Can you work these out from the model? Positions are in its coordinate system, mm. A direction names the side the tool comes from. Give positions to 0.01 mm unless a question says otherwise; leave off trailing zeros. Write each loop counter-clockwise with the first axis right and the second up, starting at its lowest first coordinate (ties: lowest second). Pieces come first, ordered by that corner, then holes.
1. On a 3-axis mill with a long thin cutter (end or side, diameter ignored), from which of +Z, -Z, +X, -X, +Y, -Y can I reach the whole of each face in a straight line? I mean faces 4 (the flat face through (-17.77, 4, 31)), 5 (the flat face through (-27.93, 4, 31)), 6 (the flat face through (-23, 1, 34.532)), 7 (the flat face through (-23, -5, 23.737)). Say none if no direction works.
2. Suppose I cut it at D-D (y = 3.81). Please give me the cut outline in (x, z).
3. Suppose I cut it at A-A (y = -4). Please give me the cut outline in (x, z), and give its area (3 significant figures).
4. Suppose I cut it at C-C (z = 28.25). Please give me the cut outline in (x, y), and give its area (3 significant figures).
5. I'm going to push flat-ended pins straight in: pin 1 (2.5 mm diameter, centred on x = -21.5, y = 5, fed in from +Z); pin 2 (1 mm diameter, centred on y = 1, z = 26, fed in from -X); pin 3 (4 mm diameter, centred on x = -21.5, y = 5, fed in from -Z); pin 4 (3 mm diameter, centred on x = -29.5, z = 23, fed in from -Y). Where does each tip first touch, or does it pass through?
6. If I drill on probe 1 along Z at (x, y) = (-15.75, -5.5); probe 2 along Y at (x, z) = (-24, 31.5); probe 3 along Y at (x, z) = (-18.5, 30.5), over which ranges is the centre line in solid material (lowest first)?
7. Suppose I cut it at B-B (x = -24). Please give me the cut outline in (y, z), and give its area (3 significant figures).
8. Thinking about a two-plate mould opening in X: for faces 1 (the flat face through (-34.915, -7, 31)), 2 (the cylindrical face through (-25.387, 3.922, 30.776)), 3 (the flat face through (-23, 1, 26.912)), which applies, pulls with the +X half, pulls with the -X half, needs draft (parallel to the pull), parting line crosses it, or undercut?
```python
from build123d import *

# Parameters (mm, degrees)
F0_W     = 24.13
F0_H     = 24.13
F1_DEPTH = 17.78
F3_DEPTH = 24.131
F4_W     = 10.16
F4_H     = 7.62
F5_DEPTH = 7.62
F6_R     = 2.54
F7_DEPTH = 15.876
F8_W     = 3.048
F8_H     = 13.97
F9_DEPTH = 24.131


with BuildPart() as f1:
    # F0 (on Front) → F1 (new body)
    with BuildSketch(Plane.XZ):
        with Locations((-22.849758, 30.722394)):
            Rectangle(F0_W, F0_H)
    extrude(amount=F1_DEPTH)

    # F2 (on face) → F3 (cut, through all)
    with BuildSketch(Plane.YZ.offset(-10.784758)):
        with BuildLine():
            Line((-17.78, 42.787394), (-17.78, 18.657394))
            ThreePointArc((-17.78, 18.657394), (-11.495566, 30.722394), (-17.78, 42.787394))
        make_face()
    extrude(amount=-F3_DEPTH, mode=Mode.SUBTRACT)

    # F4 (on face) → F5 (join)
    with BuildSketch(Plane(origin=(0, 0, 0), x_dir=(-1, 0, 0), z_dir=(0, 1, 0))):
        with Locations((22.849758, 30.722394)):
            Rectangle(F4_W, F4_H)
    extrude(amount=F5_DEPTH)

    # F6 (on face) → F7 (cut, through all)
    with BuildSketch(Plane.XY.offset(34.532394)):
        with Locations((-22.849758, 3.81)):
            Circle(F6_R)
    extrude(amount=-F7_DEPTH, mode=Mode.SUBTRACT)

    # F8 (on face) → F9 (cut, through all)
    with BuildSketch(Plane.YZ.offset(-10.784758)):
        with Locations((-4.826, 30.722394)):
            Rectangle(F8_W, F8_H)
    extrude(amount=-F9_DEPTH, mode=Mode.SUBTRACT)


solid = f1.part
```
Checks:
1. face 4: +Z, -Z, +X, +Y
1. face 5: +Z, -Z, -X, +Y
1. face 6: +Z, +X, -X, +Y
1. face 7: +X, -X
2. outline: (-27.93, 26.91) - (-25.39, 26.91) - (-25.39, 34.53) - (-27.93, 34.53) - close; (-20.31, 26.91) - (-17.77, 26.91) - (-17.77, 34.53) - (-20.31, 34.53) - close
3. outline: (-34.91, 18.66) - (-10.78, 18.66) - (-10.78, 23.74) - (-34.91, 23.74) - close; (-34.91, 37.71) - (-10.78, 37.71) - (-10.78, 42.79) - (-34.91, 42.79) - close
3. area: 245 mm2
4. outline: (-34.91, -11.7) - (-10.78, -11.7) - (-10.78, -6.35) - (-34.91, -6.35) - close; (-34.91, -3.3) - (-10.78, -3.3) - (-10.78, 0) - (-17.77, 0) - (-17.77, 7.62) - (-27.93, 7.62) - (-27.93, 0) - (-34.91, 0) - close; hole circle Ø5.08 at (-22.85, 3.81)
4. area: 266 mm2
5. pin 1: stops at z = 34.53
5. pin 2: passes through
5. pin 3: stops at z = 26.91
5. pin 4: stops at y = -14.74
6. probe 1: z = 18.66 to 23.74, 37.71 to 42.79
6. probe 2: y = -11.52 to -6.35, -3.3 to 1.55, 6.07 to 7.62
6. probe 3: y = -11.5 to -6.35, -3.3 to 7.62
7. outline: (-17.78, 18.66) - (0, 18.66) - (0, 26.91) - (1.55, 26.91) - (1.55, 34.53) - (0, 34.53) - (0, 42.79) - (-17.78, 42.79) arc R14.72 cw to start; (6.07, 26.91) - (7.62, 26.91) - (7.62, 34.53) - (6.07, 34.53) - close; hole (-6.35, 23.74) - (-3.3, 23.74) - (-3.3, 37.71) - (-6.35, 37.71) - close
7. area: 304 mm2
8. face 1: pulls with the -X half
8. face 2: undercut
8. face 3: needs draft
